Autodesk Inventor part; units mm, degrees
ref_plane "YZ Plane" through (0, 0, 0) normal (1, 0, 0) x (0, 1, 0)
ref_plane "XZ Plane" through (0, 0, 0) normal (0, 1, 0) x (-1, 0, 0)
ref_plane "XY Plane" through (0, 0, 0) normal (0, 0, 1) x (1, 0, 0)
sketch "Skizze1" plane through (0, 0, 0) normal (0, 1, 0) x (-1, 0, 0)
  line L0 (0, 0) -> (5, 0)
  line L1 (5, 0) -> (5, -85)
  line L2 (5, -85) -> (0, -85)
  line L3 (0, -85) -> (0, 0)
  line L4 (0, 0) -> (25, 0)
  line L5 (25, 0) -> (25, -5)
  line L6 (25, -5) -> (0, -5)
  line L7 (0, -5) -> (0, 0)
  line L8 (25, 0) -> (30, 0)
  line L9 (30, 0) -> (30, -85)
  line L10 (30, -85) -> (25, -85)
  line L11 (25, -85) -> (25, 0)
  line L12 (30, -85) -> (0, -85)
  line L13 (0, -85) -> (0, -80)
  line L14 (0, -80) -> (30, -80)
  line L15 (30, -80) -> (30, -85)
  point P0 (5, -5)
  point P1 (25, -80)
  point P2 (5, -80)
  dimension "d0" = 5
  dimension "d1" = 85
  dimension "d2" = 25
  dimension "d3" = 5
  dimension "d4" = 5
  dimension "d5" = 85
  dimension "d13" = 30
  dimension "d14" = 5
extrude "Extrusion1" add sketch "Skizze1" along normal blind 15 contours L0 L1 L6 L3 | L4 L5 L6 L1 | L6 L1 L14 L3 | L8 L9 L14 L11 L5 | L14 L1 L2 L3 | L14 L11 L12 L1 | L14 L9 L10 L11
fillet "Rundung1" radius 10 2 edges at (-30, 7.5, 0) (-30, 7.5, -85)
fillet "Rundung2" radius 5 2 edges at (-25, 7.5, -5) (-25, 7.5, -80)
fillet "Rundung3" radius 2 2 edges at (-5, 7.5, -5) (-5, 7.5, -80)
sketch "Skizze2" plane through (-5, 0, -75) normal (-1, 0, 0) x (0, 0, 1)
  line L0 (-10, 0) -> (-10, 15)
  line L1 (-10, 7.5) -> (75, 7.5) construction
  line L2 (75, 0) -> (75, 15) construction
  point P0 (62.5, 7.5)
  point P1 (2.5, 7.5)
  dimension "d15" = 60
  dimension "d16" = 12.5
hole "Bohrung1" at (-5, 7.5, -12.5) at (-5, 7.5, -72.5) direction (1, 0, 0) diameter 4.5 depth 5 countersink diameter 9.4 countersink angle 90
sketch "Skizze3" plane through (-30, 0, -75) normal (-1, 0, 0) x (0, 0, 1)
  circle A0 centre (2.5, 7.5) radius 4.7
  circle A1 centre (62.5, 7.5) radius 4.7
  circle A2 centre (2.5, 7.5) radius 2.25
  point P0 (75, 0)
hole "Bohrung2" at (-30, 7.5, -72.5) at (-30, 7.5, -12.5) direction (1, 0, 0) diameter 3 depth 25
chamfer "Fasen1" distance 1.5 angle 45 8 edges at (-5, 0, -42.5) (-13.5, 0, -5) (-25, 0, -42.5) (-13.5, 0, -80) (-5, 15, -42.5) (-13.5, 15, -5) (-25, 15, -42.5) (-13.5, 15, -80)
chamfer "Fasen2" distance 1.5 angle 45 10 edges at (-30, 0, -42.5) (-27.0711, 0, -2.9289) (-10, 0, 0) (-27.0711, 0, -82.0711) (-10, 0, -85) (-30, 15, -42.5) (-27.0711, 15, -2.9289) (-10, 15, 0) (-27.0711, 15, -82.0711) (-10, 15, -85)
properties part number "260_Handle"
Input: part model. Units: mm. Frame: model coordinates. A direction names the side the tool comes from. Give positions to 0.01 mm unless a question says otherwise; leave off trailing zeros. Order: outer loops, then holes, each group sorted by start corner. A loop starts at its lowest first (then second) coordinate and runs counter-clockwise, first axis right, second up. Notation, with made-up numbers: (-39.75, 9) - (-18.75, 9) arc R18 cw to (-18.75, 19) - close; hole circle Ø7 at (-8.5, 41). An arc over 180 degrees is marked (long way). One line per item, written item: value.
1. Cut plane C-C, the plane z = -12.5. Output: boundary loops of the cut face in (x, y), and give its area (3 significant figures).
Determined:
outline: (-30, 1.5) - (-28.5, 0) - (-26.5, 0) - (-25, 1.5) - (-25, 6) - (-30, 6) - close; (-30, 9) - (-25, 9) - (-25, 13.5) - (-26.5, 15) - (-28.5, 15) - (-30, 13.5) - close; (-5, 1.5) - (-3.5, 0) - (0, 0) - (0, 5.25) - (-2.55, 5.25) - (-5, 2.8) - close; (-5, 12.2) - (-2.55, 9.75) - (0, 9.75) - (0, 15) - (-3.5, 15) - (-5, 13.5) - close
area: 99.7 mm2
2. Draft query along X for faces 1 (the face through (-27.465, 8.964, -12.825)), 2 (the face through (-14, 7, -5)), 3 (the face through (-23, 8, -79)), 4 (the face through (-29.3, 14.2, -42)). Return one class per face: released by +X, released by -X, zero draft, split by the parting line, or undercut.
Determined:
face 1: zero draft
face 2: undercut
face 3: undercut
face 4: released by -X
3. Cut plane B-B, the plane y = 7.5. Give the number of separate pieces and of enclosed holes in the cut face, and give its area (3 significant figures).
Determined:
separate pieces: 4
enclosed holes: 0
area: 933 mm2
4. Line query: probe 1 along X at (y, z) = (4.25, -24); probe 2 along Z at (x, y) = (-27.55, 7.5); probe 3 along Y at (x, z) = (-27.8, -72.5). Output: solid intervals per line, ascending.
Determined:
probe 1: -30 to -25, -5 to 0
probe 2: -81.56 to -74, -71 to -14, -11 to -3.44
probe 3: 0 to 6, 9 to 15
5. Cut plane A-A, the plane x = -9. Output: boundary loops of the cut face in (y, z), and give its area (3 significant figures).
Determined:
outline: (0, -83.5) - (1.5, -85) - (13.5, -85) - (15, -83.5) - (15, -81.5) - (13.5, -80) - (1.5, -80) - (0, -81.5) - close; (0, -3.5) - (1.5, -5) - (13.5, -5) - (15, -3.5) - (15, -1.5) - (13.5, 0) - (1.5, 0) - (0, -1.5) - close
area: 141 mm2
6. Reachability of faces 5 (the face through (-5.57, 7.58, -79.4)), 6 (the face through (-26.26, 0.26, -3.87)), 7 (the face through (-4.3, 14.2, -42)), 8 (the face through (-4.2, 0.7, -43)), 9 (the face through (-2.7, 7.6, -14.9)) from +Z, -Z, +X, -X, +Y, -Y: full face, straight path, thin tool, end or side. Return the list, or none.
Determined:
face 5: +Y, -Y
face 6: +Z, -X, -Y
face 7: +Y
face 8: -Y
face 9: none
